Verification items for the finished model (mm, model axes). A direction names the side the tool comes from. Round coordinates to 2 decimals unless told otherwise and drop trailing zeros. Write each loop counter-clockwise with the first axis right and the second up, starting at its lowest first coordinate (ties: lowest second). Pieces come first, ordered by that corner, then holes. Notation, with made-up numbers: (44.25, -14) - (94.25, -14) arc R17 cw to (94.25, 18) - close; hole circle Ø11 at (66.25, 29). An arc over 180 degrees is marked (long way). Answer as a JSON object with one key per item and string values.
```python
from build123d import *

# Parameters (mm, degrees)
SCHIZZO1_R                  = 72.5
ESTRUSIONE1_DEPTH           = 10
SCHIZZO2_R                  = 19.5
ESTRUSIONE2_DEPTH           = 26
ESTRUSIONE5_DEPTH           = 62
ESTRUSIONE5_DEPTH_BACK      = 5
SCHIZZO5_R                  = 15
SMUSSO2_SIZE                = 1
RACCORDO1_R                 = 1
ESTRUSIONE3_DEPTH           = 5
RIPETIZIONECIRCOLARE1_COUNT = 4
SMUSSO3_SIZE                = 1
M10_GIOCHI_FORO1_D          = 11


with BuildPart() as part:
    # Schizzo1 → Estrusione1 (new body)
    with BuildSketch(Plane.XY):
        Circle(SCHIZZO1_R)
    extrude(amount=ESTRUSIONE1_DEPTH)

    # Schizzo2 → Estrusione2 (add)
    with BuildSketch(Plane.XY.offset(10)):
        with Locations(Location((0, 0, 0), (0, 0, 180))):
            Circle(SCHIZZO2_R)
    extrude(amount=ESTRUSIONE2_DEPTH)

    # Schizzo5 → Estrusione5 (add, two sides: drawn at the far end of the back side and taken through both)
    with BuildSketch(Plane.XY.offset(36).offset(-ESTRUSIONE5_DEPTH_BACK)):
        Circle(SCHIZZO5_R)
    extrude(amount=ESTRUSIONE5_DEPTH + ESTRUSIONE5_DEPTH_BACK)

    # Smusso2
    smusso2_edges = [part.edges().sort_by_distance(p)[0] for p in [
        (-72.5, 0, 10),
    ]]
    chamfer(smusso2_edges, length=SMUSSO2_SIZE)

    # Raccordo1
    raccordo1_edges = [part.edges().sort_by_distance(p)[0] for p in [
        (19.5, 0, 10),
    ]]
    fillet(raccordo1_edges, radius=RACCORDO1_R)

    # Schizzo3 → Estrusione3 (cut)
    with BuildSketch(Plane(origin=(0, 0, 0), x_dir=(-1, 0, 0), z_dir=(0, 0, -1))):
        with BuildLine():
            Line((-57.271310306, 44.454999897), (-23.243993136, 11.87294332))
            ThreePointArc((-23.243993136, 11.87294332), (-12.639887246, 12.103026498), (-12.869970423, 22.707132388))
            Line((-12.869970423, 22.707132388), (-46.897287593, 55.289188965))
            ThreePointArc((-46.897287593, 55.289188965), (-52.365247161, 50.141109778), (-57.271310306, 44.454999897))
        make_face()
    estrusione3 = extrude(amount=-ESTRUSIONE3_DEPTH, mode=Mode.SUBTRACT)

    # RipetizioneCircolare1: Estrusione3 ×4 about axis
    ripetizionecircolare1_axis = Axis((0, 0, 0), (0, 0, 1))
    for i in range(1, RIPETIZIONECIRCOLARE1_COUNT):
        add(estrusione3.rotate(ripetizionecircolare1_axis, i * 360 / RIPETIZIONECIRCOLARE1_COUNT), mode=Mode.SUBTRACT)

    # Smusso3
    smusso3_edges = [part.edges().sort_by_distance(p)[0] for p in [
        (-15, 0, 98),
    ]]
    chamfer(smusso3_edges, length=SMUSSO3_SIZE)

    # M10 Giochi foro1 (through all)
    with Locations(Plane(origin=(8.775277543, -26.129129274, 10), x_dir=(0.9999999999861032, 5.271953212239764e-06, 0), z_dir=(0, 0, 1))):
        with Locations((-8.776166907, 82.129175527), (-8.776166907, -29.870824473), (-64.776166907, 26.129175527), (47.223833093, 26.129175527)):
            Hole(M10_GIOCHI_FORO1_D / 2)


solid = part.part
```
Q1. Gauge pin test, flat ends, axial feed: P1, Ø3, axis at x = 47, y = 7.5, coming from the +Z side; P2, Ø9, axis at x = 0, y = -56, coming from the -Z side. Record the tip position at first contact, or that the pin passes through.
Geometry check:
{"P1": "stops at z = 10", "P2": "passes through"}
Q2. Set-up check for faces 1 (the cylindrical face through (-50.506, 0.242, 4.93)), 2 (the flat face through (-40.496, -28.392, 2.465)): record each of +Z, -Z, +X, -X, +Y, -Y from which the full face is reachable in a straight line by a thin tool's end or side.
Geometry check:
{"face 1": "+Z, -Z", "face 2": "-Z"}
Q3. Material ranges on line 1 along Z through (x, y) = (36, 20); line 2 along Y through (x, z) = (56, 7), recorded low to high. Write a range as [from, to].
Geometry check:
{"line 1": "z = [0, 10]", "line 2": "y = [-46.05, -5.5], [5.5, 46.05]"}
Q4. Release check for a two-part mould opening along Y. For faces 3 (the flat face through (38.77, -29.645, 2.465)), 4 (the flat face through (0, 0, 98)), 5 (the cylindrical face through (33.45, -64.32, 4.44)) record: released by +Y, released by -Y, zero draft, split by the parting line, or undercut.
Geometry check:
{"face 3": "undercut", "face 4": "zero draft", "face 5": "split by the parting line"}
Q5. Section check B-B, the plane z = 68.5. Record the cut outline in (x, y).
Geometry check:
{"outline": "circle Ø30 at (0, 0)"}
Q6. Section check A-A, the plane x = 0. Record the cut outline in (y, z).
Geometry check:
{"outline": "(-72.5, 0) - (-61.5, 0) - (-61.5, 10) - (-71.5, 10) - (-72.5, 9) - close; (-50.5, 0) - (50.5, 0) - (50.5, 10) - (20.5, 10) arc R1 cw to (19.5, 11) - (19.5, 36) - (15, 36) - (15, 97) - (14, 98) - (-14, 98) - (-15, 97) - (-15, 36) - (-19.5, 36) - (-19.5, 11) arc R1 cw to (-20.5, 10) - (-50.5, 10) - close; (61.5, 0) - (72.5, 0) - (72.5, 9) - (71.5, 10) - (61.5, 10) - close"}
